Autodesk Inventor part; units mm, degrees
ref_plane "YZ Plane" through (0, 0, 0) normal (1, 0, 0) x (0, 1, 0)
ref_plane "XZ Plane" through (0, 0, 0) normal (0, 1, 0) x (-1, 0, 0)
ref_plane "XY Plane" through (0, 0, 0) normal (0, 0, 1) x (1, 0, 0)
sketch "Sketch1" plane through (0, 0, 0) normal (1, 0, 0) x (0, 1, 0)
  line L0 (-44.45, 222.25) -> (44.45, 222.25)
  line L1 (44.45, 222.25) -> (44.45, -222.25)
  line L2 (44.45, -222.25) -> (-44.45, -222.25)
  line L3 (-44.45, -222.25) -> (-44.45, 222.25)
  line L4 (-44.45, 222.25) -> (44.45, -222.25) construction
  line L5 (44.45, 222.25) -> (-44.45, -222.25) construction
  point P0 (0, 0)
  dimension "d0" = 88.9
  dimension "d1" = 444.5
extrude "Extrusion1" add sketch "Sketch1" along normal blind 6.35
sketch "Sketch2" plane through (0, 0, 0) normal (-1, 0, 0) x (0, 0, 1)
  line L0 (-222.25, -44.45) -> (-222.25, 44.45)
  line L1 (-222.25, 44.45) -> (-209.55, 44.45)
  line L2 (-209.55, 44.45) -> (-209.55, 38.1)
  line L3 (-209.55, 38.1) -> (-222.25, 38.1)
  line L4 (-222.25, 38.1) -> (-222.25, 44.45)
  line L5 (-222.25, 44.45) -> (222.25, 44.45)
  line L6 (222.25, 44.45) -> (209.55, 44.45)
  line L7 (209.55, 44.45) -> (209.55, 38.1)
  line L8 (209.55, 38.1) -> (222.25, 38.1)
  line L9 (222.25, 38.1) -> (222.25, 44.45)
  line L10 (222.25, -44.45) -> (-222.25, -44.45)
  line L11 (-101.6, -44.45) -> (-88.9, -44.45)
  line L12 (-88.9, -44.45) -> (-88.9, -38.1)
  line L13 (-88.9, -38.1) -> (-101.6, -38.1)
  line L14 (-101.6, -38.1) -> (-101.6, -44.45)
  line L15 (88.9, -44.45) -> (101.6, -44.45)
  line L16 (101.6, -44.45) -> (101.6, -38.1)
  line L17 (101.6, -38.1) -> (88.9, -38.1)
  line L18 (88.9, -38.1) -> (88.9, -44.45)
  point P0 (0, 0)
  dimension "d4" = 12.7
  dimension "d5" = 6.35
  dimension "d6" = 6.35
  dimension "d7" = 12.7
  dimension "d8" = 6.35
  dimension "d9" = 12.7
  dimension "d10" = 12.7
  dimension "d11" = 88.9
  dimension "d12" = 88.9
extrude "Extrusion2" add sketch "Sketch2" along normal blind 6.35
sketch "Sketch3" plane through (6.35, 44.45, 222.25) normal (0, 1, 0) x (1, 0, 0)
  line L0 (-6.35, 120.65) -> (-6.35, 0)
  line L1 (0, 0) -> (-12.7, 0)
  line L2 (-12.7, 431.8) -> (-12.7, 444.5)
  line L3 (0, 444.5) -> (-12.7, 444.5)
  line L4 (-6.35, 431.8) -> (-12.7, 431.8)
  line L5 (-6.35, 12.7) -> (-12.7, 12.7)
  line L6 (-12.7, 0) -> (-12.7, 12.7)
  point P0 (-6.35, 222.25)
  point P1 (-9.525, 6.35)
  point P2 (-9.525, 438.15)
  dimension "d44" = 3.175
  dimension "d45" = 6.35
  dimension "d46" = 6.35
  dimension "d47" = 3.175
sketch "Sketch4" plane through (6.35, -44.45, -222.25) normal (0, -1, 0) x (1, 0, 0)
  line L0 (-6.35, 311.15) -> (-6.35, 323.85)
  line L1 (-6.35, 431.8) -> (-6.35, 12.7)
  line L2 (-6.35, 120.65) -> (-12.7, 120.65)
  line L3 (-12.7, 120.65) -> (-12.7, 133.35)
  line L4 (-12.7, 311.15) -> (-12.7, 323.85)
  line L5 (-6.35, 323.85) -> (-12.7, 323.85)
  point P0 (-6.35, 222.25)
  point P1 (-9.525, 317.5)
  point P2 (-9.525, 127)
  dimension "d33" = 3.175
  dimension "d34" = 6.35
  dimension "d35" = 3.175
  dimension "d36" = 6.35
hole "Hole3" at (-3.175, -44.45, 95.25) at (-3.175, -44.45, -95.25) direction (0, 1, 0) diameter 5.08 depth 6.35 tip angle 118
hole "Hole4" at (-3.175, 44.45, 215.9) at (-3.175, 44.45, -215.9) direction (0, -1, 0) diameter 5.08 depth 6.35 tip angle 118
equation "\"d6\" = d5"
equation "\"d7\" = d4"
equation "\"d8\" = d5"
equation "\"d9\" = d4"
equation "\"d10\" = d9"
equation "\"d42\" = d15"
equation "\"d53\" = d15"
equation "\"d15\" = d17"
equation "\"d17\" = d16"
properties part number "FrameTestinsidePlate"
Design review of the part built by this model. Coordinates are the model's own, in mm. Coordinates: 2 decimals unless noted, no trailing zeros. Order: outer loops, then holes, each group sorted by start corner. A loop starts at its lowest first (then second) coordinate and runs counter-clockwise, first axis right, second up. Notation, with made-up numbers: (47.5, -11) -> (82.5, -11) arc R9 cw to (82.5, -5) -> close; hole circle Ø8 at (-24.5, -10.5). An arc over 180 degrees is marked (long way). One line per item, written item: value.
1) Clearance check with flat-ended pins moving along their axes: P1, Ø1.9, axis at x = -4.5, z = 98, coming from the +Y side; P2, Ø3, axis at x = -4, y = -40, coming from the -Z side; P3, Ø5, axis at x = -4.5, y = -42.5, coming from the +Z side. State where each tip first meets the part, or that it passes through.
Output values:
P1: stops at y = -38.1
P2: stops at z = -101.6
P3: stops at z = 101.6
2) We need section A-A, the plane y = 12. Give the boundary of the cut face in (x, z), then the cut area to 3 significant figures.
Output values:
outline: (0, -222.25) -> (6.35, -222.25) -> (6.35, 222.25) -> (0, 222.25) -> close
area: 2,820 mm2
3) We need section B-B, the plane z = 71. Give the boundary of the cut face in (x, y).
Output values:
outline: (0, -44.45) -> (6.35, -44.45) -> (6.35, 44.45) -> (0, 44.45) -> close
4) To check wall thickness, follow probe 1 along X at (y, z) = (43, 215.9) (3 decimals); probe 2 along X at (y, z) = (35, -17). State the ranges of each line that lie inside material, in increasing order. Write a range as [from, to].
Output values:
probe 1: x = [-6.35, -5.715], [-0.635, 6.35]
probe 2: x = [0, 6.35]
